from build123d import *

# Parameters (mm, degrees)
BOSS_EXTRU_1_OUTLINE_R  = 2.2
BOSS_EXTRU_1_DEPTH      = 5
ESQUISSE3_W             = 5
ESQUISSE3_H             = 5
BOSS_EXTRU_3_DEPTH      = 5
ESQUISSE4_W             = 3
ESQUISSE4_H             = 3
ENL_V_MAT_EXTRU_1_DEPTH = 10
ESQUISSE6_W             = 13
ESQUISSE6_H             = 5.8
ENL_V_MAT_EXTRU_2_DEPTH = 10
ESQUISSE7_W             = 5.8
ESQUISSE7_H             = 13
ENL_V_MAT_EXTRU_3_DEPTH = 10


# Read off the part's stored shape, not the designer's step: Boss.-Extru.1
with BuildPart() as part:
    # Boss.-Extru.1 outline → Boss.-Extru.1 (new body)
    with BuildSketch(Plane(origin=(0, 0, 0), x_dir=(0, 0, -1), z_dir=(1, 0, 0))):
        Polygon((-12.5, 40.000001465), (-17.5, 40.000001465), (-17.5, -40.000001465), (-12.5, -40.000001465), (-12.5, -35.000001465), (-7.5, -35.000001465), (-7.5, -40.000001465), (-2.5, -40.000001465), (-2.5, -35.000001465), (2.5, -35.000001465), (2.5, -40.000001465), (7.5, -40.000001465), (7.5, -35.000001465), (12.5, -35.000001465), (12.5, -40.000001465), (17.5, -40.000001465), (17.5, 40.000001465), (12.5, 40.000001465), (12.5, 35.000001047), (7.5, 35.000000628), (7.5, 40.000001465), (2.5, 40.000001465), (2.5, 35.000000209), (-2.5, 34.999999791), (-2.5, 40.000001465), (-7.5, 40.000001465), (-7.5, 34.999999372), (-12.5, 34.999998953), align=None)
        with Locations((-7.5, 14.999999372)):
            Circle(BOSS_EXTRU_1_OUTLINE_R, mode=Mode.SUBTRACT)
    extrude(amount=BOSS_EXTRU_1_DEPTH)

    # Esquisse3 → Boss.-Extru.3 (add)
    with BuildSketch(Plane(origin=(0, 40.000001465, 0), x_dir=(1, 0, 0), z_dir=(0, 1, 0))):
        with Locations((2.5, -15)):
            Rectangle(ESQUISSE3_W, ESQUISSE3_H)
        with Locations((2.5, -5)):
            Rectangle(ESQUISSE3_W, ESQUISSE3_H)
        with Locations((2.5, 5)):
            Rectangle(ESQUISSE3_W, ESQUISSE3_H)
        with Locations((2.5, 15)):
            Rectangle(ESQUISSE3_W, ESQUISSE3_H)
    extrude(amount=BOSS_EXTRU_3_DEPTH)

    # Esquisse4 → Enlèv. mat.-Extru.1 (cut)
    with BuildSketch(Plane.ZY):
        with Locations((-3, -4.5)):
            Rectangle(ESQUISSE4_W, ESQUISSE4_H)
        with Locations((-9, -4.5)):
            Rectangle(ESQUISSE4_W, ESQUISSE4_H)
        with Locations((3, -4.5)):
            Rectangle(ESQUISSE4_W, ESQUISSE4_H)
        with Locations((9, -4.5)):
            Rectangle(ESQUISSE4_W, ESQUISSE4_H)
        with Locations((9, 4.5)):
            Rectangle(ESQUISSE4_W, ESQUISSE4_H)
        with Locations((3, 4.5)):
            Rectangle(ESQUISSE4_W, ESQUISSE4_H)
        with Locations((-3, 4.5)):
            Rectangle(ESQUISSE4_W, ESQUISSE4_H)
        with Locations((-9, 4.5)):
            Rectangle(ESQUISSE4_W, ESQUISSE4_H)
    extrude(amount=-ENL_V_MAT_EXTRU_1_DEPTH, mode=Mode.SUBTRACT)

    # Esquisse6 → Enlèv. mat.-Extru.2 (cut)
    with BuildSketch(Plane.ZY):
        with Locations((0, -17.1)):
            Rectangle(ESQUISSE6_W, ESQUISSE6_H)
    extrude(amount=-ENL_V_MAT_EXTRU_2_DEPTH, mode=Mode.SUBTRACT)

    # Esquisse7 → Enlèv. mat.-Extru.3 (cut)
    with BuildSketch(Plane.ZY):
        with Locations((-13.8, 26.5)):
            Rectangle(ESQUISSE7_W, ESQUISSE7_H)
        with Locations((13.8, 26.5)):
            Rectangle(ESQUISSE7_W, ESQUISSE7_H)
    extrude(amount=-ENL_V_MAT_EXTRU_3_DEPTH, mode=Mode.SUBTRACT)


solid = part.part
Build history of the part. All positions in model axes, mm. A direction names the side the tool comes from. Round coordinates to 2 decimals unless told otherwise and drop trailing zeros. Write each loop counter-clockwise with the first axis right and the second up, starting at its lowest first coordinate (ties: lowest second). Pieces come first, ordered by that corner, then holes. Notation, with made-up numbers: M 10,-30 L 14,-30 A18 cw 14,-14 Z; hole C -2.75,17 d4. An arc over 180 degrees is marked long. Answer in a Markdown table with one row per item.
1. Saw through at C-C (x = 2.6). State how many separate pieces and enclosed holes the cut face has, and give its area (3 significant figures).
Geometry check:
| item | result |
|---|---|
| separate pieces | 1 |
| enclosed holes | 12 |
| area | 2,440 mm2 |
2. Saw through at B-B (y = 15). List the corners of the cut face in (x, z), and give its area (3 significant figures).
Geometry check:
| item | result |
|---|---|
| outline | M 0,-17.5 L 5,-17.5 L 5,5.3 L 0,5.3 Z; M 0,9.7 L 5,9.7 L 5,17.5 L 0,17.5 Z |
| area | 153 mm2 |
3. Mould opens along Z. For faces 5 (the face through (2, 4, 1.5)), 6 (the face through (2, 2, -17.5)), 7 (the face through (5, 2, 0)) say: +Z half, -Z half, draft (parallel to the pull), parting line (faces both ways), or undercut.
Geometry check:
| item | result |
|---|---|
| face 5 | undercut |
| face 6 | -Z half |
| face 7 | draft |
4. Flat gauge pin, fed straight in: P1, Ø0.9, axis at x = 2.5, z = 8.5, coming from the +Y side. Where does the tip first touch, or does it go through?
Geometry check:
| item | result |
|---|---|
| P1 | y = 35 |
5. Saw through at A-A (z = 14). List the corners of the cut face in (x, y).
Geometry check:
| item | result |
|---|---|
| outline | M 0,-40 L 5,-40 L 5,20 L 0,20 Z; M 0,33 L 5,33 L 5,45 L 0,45 Z |
6. Which spindle directions (+Z, -Z, +X, -X, +Y, -Y) get a long thin tool onto all of the face, cutting with end or side? Do faces 1 (the face through (2, 40, -12.5)), 2 (the face through (2, 6, 3)), 3 (the face through (2, -40, -15)), 4 (the face through (2, -35, 0)). Say none if no direction does.
Geometry check:
| item | result |
|---|---|
| face 1 | +X, -X, +Y |
| face 2 | +X, -X |
| face 3 | +Z, -Z, +X, -X, -Y |
| face 4 | +X, -X, -Y |
7. Probe L1, parallel to Y at x = 2.1, z = 4; L2, parallel to Y at x = 2.1, z = -8; L3, parallel to Y at x = 2.4, z = -2. List the from-to ranges inside material, lowest first. Write a range as [from, to].
Geometry check:
| item | result |
|---|---|
| L1 | [-40, -20], [-14.2, -6], [-3, 3], [6, 45] |
| L2 | [-35, -6], [-3, 3], [6, 35] |
| L3 | [-35, -20], [-14.2, -6], [-3, 3], [6, 35] |
